```python
from build123d import *

# Parameters (mm, degrees)
F1_DEPTH = 150
F3_DEPTH = 188
F4_R     = 45
F5_R     = 15
F6_DEPTH = 133
F7_R     = 15
F8_DEPTH = 179


with BuildPart() as f1:
    # F0 (on Front) → F1 (new body)
    with BuildSketch(Plane.XZ):
        Polygon((-50, 0), (0, 0), (50, 0), (50, -75), (75, -75), (75, 245), (49.5, 245), (49.5, 375), (-49.5, 375), (-49.5, 245), (-75, 245), (-75, -75), (-50, -75), align=None)
    extrude(amount=F1_DEPTH)

    # F2 (on face) → F3 (cut)
    with BuildSketch(Plane.YZ.offset(75)):
        Polygon((-50, 50), (-50, -75), (0, -75), (0, 125), align=None)
    extrude(amount=-F3_DEPTH, mode=Mode.SUBTRACT)

    # F4
    f4_edges = [f1.edges().sort_by_distance(p)[0] for p in [
        (0, -150, 375),
        (0, 0, 375),
    ]]
    fillet(f4_edges, radius=F4_R)

    # F5 (on face) → F6 (cut)
    with BuildSketch(Plane.YZ.offset(49.5)):
        with Locations((-75, 345)):
            Circle(F5_R)
    extrude(amount=-F6_DEPTH, mode=Mode.SUBTRACT)

    # F7 (on face) → F8 (cut)
    with BuildSketch(Plane.YZ.offset(75)):
        with Locations((-100, -50)):
            Circle(F7_R)
    extrude(amount=-F8_DEPTH, mode=Mode.SUBTRACT)


solid = f1.part
```
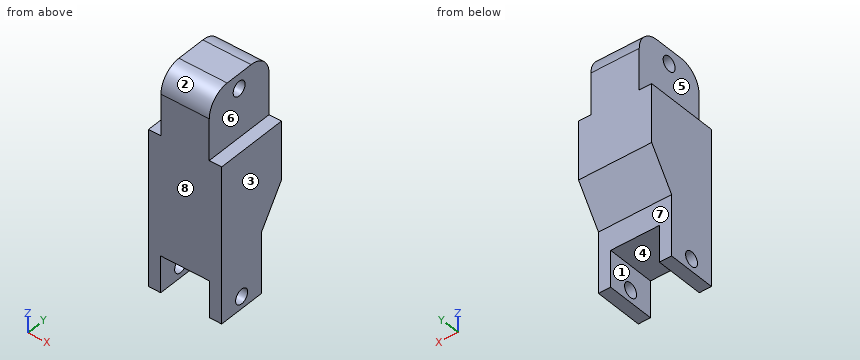
Read the model definition and answer for the solid it produces. Units are mm, in the model's axes. Face numbers are marked on the shaded views. A direction names the side the tool comes from. Give positions to 0.01 mm unless a question says otherwise; leave off trailing zeros. Write each loop counter-clockwise with the first axis right and the second up, starting at its lowest first coordinate (ties: lowest second). Pieces come first, ordered by that corner, then holes. Notation, with made-up numbers: (7, 24.25) -> (21, 24.25) arc R7 cw to (21, 29.25) -> close; hole circle Ø5 at (13.25, -13.75). An arc over 180 degrees is marked (long way). Answer in a Markdown table with one row per item.
1) Straight lines are drawn through the part: line 1 (Z direction, x = -65.5, y = -100); line 2 (X direction, y = -131, z = -9); line 3 (Z direction, x = -30, y = -75). For each, find the intervals that lie inside material, in ascending order. Write a range as [from, to].
Results list:
| item | result |
|---|---|
| line 1 | [-75, -65], [-35, 245] |
| line 2 | [-75, -50], [50, 75] |
| line 3 | [0, 330], [360, 375] |
2) Section C-C on y = -100 is taken. Give the vertices of the cut face in (x, z).
Results list:
| item | result |
|---|---|
| outline | (-75, -75) -> (-50, -75) -> (-50, -65) -> (-75, -65) -> close; (-75, -35) -> (-50, -35) -> (-50, 0) -> (50, 0) -> (50, -35) -> (75, -35) -> (75, 245) -> (49.5, 245) -> (49.5, 375) -> (-49.5, 375) -> (-49.5, 245) -> (-75, 245) -> close; (50, -75) -> (75, -75) -> (75, -65) -> (50, -65) -> close |
3) Section B-B on z = -50 is taken. Give the vertices of the cut face in (x, y), plus the area to 3 significant figures.
Results list:
| item | result |
|---|---|
| outline | (-75, -150) -> (-50, -150) -> (-50, -115) -> (-75, -115) -> close; (-75, -85) -> (-50, -85) -> (-50, -50) -> (-75, -50) -> close; (50, -150) -> (75, -150) -> (75, -115) -> (50, -115) -> close; (50, -85) -> (75, -85) -> (75, -50) -> (50, -50) -> close |
| area | 3,500 mm^2 |
4) Section A-A on x = 31 is taken. Give the vertices of the cut face in (y, z).
Results list:
| item | result |
|---|---|
| outline | (-150, 0) -> (-50, 0) -> (-50, 50) -> (0, 125) -> (0, 330) arc R45 ccw to (-45, 375) -> (-105, 375) arc R45 ccw to (-150, 330) -> close; hole circle Ø30 at (-75, 345) |
5) Each of these flat-tipped pins is pushed along its axis until it touches: pin 1 Ø12 at (x, y) = (25, -100) entering from -Z; pin 2 Ø12 at (y, z) = (-61.5, 267.5) entering from +X; pin 3 Ø2 at (x, z) = (2, 118.5) entering from +Y. Where does it stop, or does it pass through?
Results list:
| item | result |
|---|---|
| pin 1 | z = 0 |
| pin 2 | x = 49.5 |
| pin 3 | y = -3.67 |
6) A tool of negligible diameter and unlimited length cuts with its end or side. For the marked faces 5, 6, 7 and 8, from which of +Z, -Z, +X, -X, +Y, -Y can it reach the whole face along a straight path? Write none if from no direction.
Results list:
| item | result |
|---|---|
| face 5 | +Z, -X, +Y, -Y |
| face 6 | +Z, +X, +Y, -Y |
| face 7 | -Z, +X, -X, +Y |
| face 8 | +Z, -Z, +X, -X, -Y |
7) Section D-D on y = -75 is taken. Give the vertices of the cut face in (x, z).
Results list:
| item | result |
|---|---|
| outline | (-75, -75) -> (-50, -75) -> (-50, 0) -> (50, 0) -> (50, -75) -> (75, -75) -> (75, 245) -> (49.5, 245) -> (49.5, 330) -> (-49.5, 330) -> (-49.5, 245) -> (-75, 245) -> close; (-49.5, 360) -> (49.5, 360) -> (49.5, 375) -> (-49.5, 375) -> close |
8) Determine the mould class of the marked faces 1, 2, 3 and 4 for opening direction X: released by +X, released by -X, zero draft, split by the parting line, or undercut.
Results list:
| item | result |
|---|---|
| face 1 | undercut |
| face 2 | zero draft |
| face 3 | released by +X |
| face 4 | undercut |
